```python
from build123d import *

# Parameters (mm, degrees)
CYLINDER907_R             = 1.5
CYLINDER907_DEPTH         = 7.35
CYLINDER903_W             = 9
CYLINDER903_H             = 1
CYLINDER903_ANGLE         = 180
CYLINDER904_W             = 11
CYLINDER904_H             = 1
CYLINDER904_ANGLE         = 180
CYLINDER906_R             = 3
CYLINDER906_DEPTH         = 7.35
CYLINDER905_R             = 4.5
CYLINDER905_DEPTH         = 1
FILLET015_R               = 5
FILLET016_R               = 0.99
FILLET016_PLACEMENT_ANGLE = 205.5


with BuildPart() as cylinder1030:
    # Cylinder907 → Cylinder907 (new body)
    with BuildSketch(Plane(origin=(0, 13.5, -0.35), x_dir=(1, 0, 0), z_dir=(0, 0, 1))):
        Circle(CYLINDER907_R)
    extrude(amount=CYLINDER907_DEPTH)


with BuildPart() as cylinder1026:
    # Cylinder903 → Cylinder903 (revolve)
    with BuildSketch(Plane.XZ):
        with Locations((4.5, 0.5)):
            Rectangle(CYLINDER903_W, CYLINDER903_H)
    revolve(axis=Axis((0, 0, 0), (0, 0, 1)), revolution_arc=CYLINDER903_ANGLE)


with BuildPart() as cut014023:
    # Cylinder904 → Cylinder904 (revolve)
    with BuildSketch(Plane.XZ):
        with Locations((5.5, 0.5)):
            Rectangle(CYLINDER904_W, CYLINDER904_H)
    revolve(axis=Axis((0, 0, 0), (0, 0, 1)), revolution_arc=CYLINDER904_ANGLE)

    # Cut014023: cut Cylinder1026
    add(cylinder1026.part, mode=Mode.SUBTRACT)


with BuildPart() as cylinder1029:
    # Cylinder906 → Cylinder906 (new body)
    with BuildSketch(Plane(origin=(0, 13.5, -0.35), x_dir=(1, 0, 0), z_dir=(0, 0, 1))):
        Circle(CYLINDER906_R)
    extrude(amount=CYLINDER906_DEPTH)


with BuildPart() as selector:
    # Cylinder905 → Cylinder905 (new body)
    with BuildSketch(Plane(origin=(0, 13.5, 0), x_dir=(1, 0, 0), z_dir=(0, 0, 1))):
        Circle(CYLINDER905_R)
    extrude(amount=CYLINDER905_DEPTH)

    # Fusion060: union Cut014023, Cylinder1029
    add(cut014023.part)
    add(cylinder1029.part)

    # Cut014024: cut Cylinder1030
    add(cylinder1030.part, mode=Mode.SUBTRACT)

    # Fillet015
    fillet015_edges = [selector.edges().sort_by_distance(p)[0] for p in [
        (-3.337446, 10.481481, 0.5),
        (3.337446, 10.481481, 0.5),
    ]]
    fillet(fillet015_edges, radius=FILLET015_R)

    # Fillet016
    fillet016_edges = [selector.edges().sort_by_distance(p)[0] for p in [
        (-11, 0, 0.5),
        (-9, 0, 0.5),
        (11, 0, 0.5),
        (9, 0, 0.5),
    ]]
    fillet(fillet016_edges, radius=FILLET016_R)


with BuildPart() as selector_1:
    # Fillet016 placement: moved
    add(selector.part.moved(Location((0.213923, -0.468228, 14.5))).rotate(Axis((0.213923, -0.468228, 14.5), (0, 0, 1)), FILLET016_PLACEMENT_ANGLE))


solid = selector_1.part
```
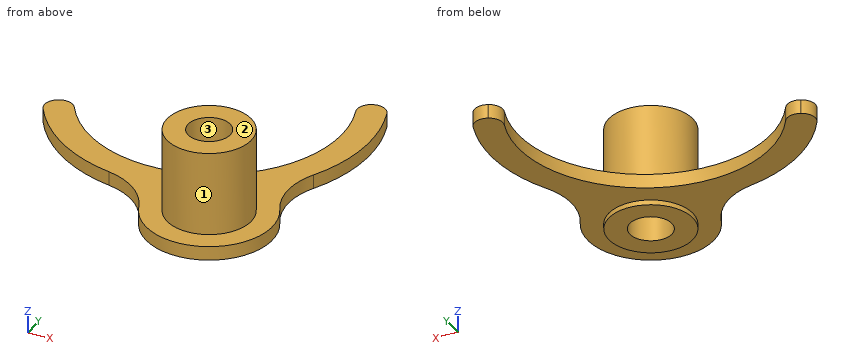
Could you check a few things on this model? Use its own coordinates, in mm. Face numbers are marked on the shaded views. Coordinates: 2 decimals unless noted, no trailing zeros. Write each loop counter-clockwise with the first axis right and the second up, starting at its lowest first coordinate (ties: lowest second). Pieces come first, ordered by that corner, then holes. Notation, with made-up numbers: (-26.5, 15.25) -> (-0.5, 15.25) arc R22 ccw to (-0.5, 29.25) -> close; hole circle Ø2 at (82.5, -26). An arc over 180 degrees is marked (long way). One line per question, with ' | ' between items. Start each with the question number.
1. If we section it at C-C (x = -5.5): Please give me the cut outline in (y, z).
2. If we section it at A-A (y = -0.75): Please give me the cut outline in (x, z), and give its area (3 significant figures).
3. Thinking about a two-plate mould opening in Y: for the marked faces 1, 2 and 3, which applies, pulls with the +Y half, pulls with the -Y half, needs draft (parallel to the pull), parting line crosses it, or undercut?
4. Will these pins go through, and if not, where does the flat tip stop? P1, Ø6, axis at x = -7, y = 0, coming from the +Z side; P2, Ø4, axis at x = -5, y = -9.5, coming from the -Z side; P3, Ø2, axis at y = -9, z = 16, coming from the +X side; P4, Ø4, axis at y = 0, z = 17, coming from the -X side.
5. Please list where these lines run through material, in increasing order: line 1 along Y through (x, z) = (6.75, 16); line 2 along Y through (x, z) = (5, 20); line 3 along Z through (x, y) = (2, -12.75).
6. If we section it at B-B (z = 16.5): Please give me the cut outline in (x, y).
Return value:
1) outline: (-9.87, 14.5) -> (-7.42, 14.5) -> (-7.42, 15.5) -> (-9.87, 15.5) -> close
2) outline: (9.21, 14.5) -> (11.21, 14.5) -> (11.21, 15.5) -> (9.21, 15.5) -> close | area: 2.00 mm²
3) face 1: parting line crosses it | face 2: needs draft | face 3: undercut
4) P1: passes through | P2: stops at z = 14.5 | P3: stops at x = 9.67 | P4: stops at x = 9.03
5) line 1: y = -15.56 to -13.97, -11.34 to -9.74 | line 2: y = -15.47 to -13.75, -11.56 to -9.83 | line 3: z = 14.5 to 15.5
6) outline: circle Ø6 at (6.03, -12.65); hole circle Ø3 at (6.03, -12.65)
